Read the model definition and answer for the solid it produces. Units are mm, in the model's axes. A direction names the side the tool comes from. Round coordinates to 2 decimals unless told otherwise and drop trailing zeros. Write each loop counter-clockwise with the first axis right and the second up, starting at its lowest first coordinate (ties: lowest second). Pieces come first, ordered by that corner, then holes. Notation, with made-up numbers: (55, 0) - (109, 0) arc R26 cw to (109, 24) - close; hole circle Ø9 at (89.25, 45). An arc over 180 degrees is marked (long way). Answer as CSV lines item,"result". Start each with the question number.
1) Each of these flat-tipped pins is pushed along its axis until it touches: pin 1 (3 mm diameter, centred on x = -393, y = -7, fed in from -Z); pin 2 (5 mm diameter, centred on x = -390.5, y = -6.5, fed in from +Z); pin 3 (4 mm diameter, centred on x = -401.69, z = 27.68, fed in from -Y). Where does it stop, or does it pass through?
2) Find section B-B on y = 2. Determine the outline of the cut face in (x, z).
3) Consider line 1 along Z through (x, y) = (-394, -3.25); line 2 along X through (y, z) = (-7.75, 81.5); line 3 along Z through (x, y) = (-392.5, 2.25). Determine where each line is inside the solid, lowest interval first.
4) Which of the six approach directions +Z, -Z, +X, -X, +Y, -Y give full straight-line access (tool end or side, diameter ignored) to faces 4 (the flat face through (-402, -11, 69)), 5 (the flat face through (-392, -4, 70.38)), 6 (the cylindrical face through (-394.09, -10.4, 34.45)), 7 (the flat face through (-397, 1, 32.678)), 8 (the flat face through (-402, -4, 32.678))?
5) Find section C-C on y = -6.5. State how many separate pieces and enclosed holes the cut face has, then the cut area to 3 significant figures.
6) For a pull along X with two mould halves and no side action, classify faces 1 (the flat face through (-404.69, 1, 58)), 2 (the cylindrical face through (-389.942, 1.479, 28.218)), 3 (the flat face through (-397, 0, 89)) as +X half, -X half, draft (parallel to the pull), parting line (faces both ways), or undercut.
7) Find section A-A on z = 69.5. Determine the outline of the cut face in (x, y).
Autodesk Inventor part; units mm, degrees
ref_plane "工作平面4" through (-396.6746, 0, 58.7787) normal (1, 0, 0) x (0, 0, -1)
ref_plane "YZ Plane" through (0, 0, 0) normal (1, 0, 0) x (0, 1, 0)
ref_plane "XZ Plane" through (0, 0, 0) normal (0, 1, 0) x (-1, 0, 0)
sketch "草圖1" plane through (0, 0, 0) normal (0, 1, 0) x (-1, 0, 0)
  line L0 (403.4401, 81.3797) -> (399.9401, 81.3797) construction
  line L1 (399.9401, 81.3797) -> (399.9401, 70.3797) construction
  line L2 (399.9401, 70.3797) -> (403.4401, 70.3797) construction
  line L3 (403.4401, 70.3797) -> (403.4401, 81.3797) construction
  line L4 (403.4401, 81.3797) -> (399.9401, 70.3797) construction
  line L5 (399.9401, 81.3797) -> (403.4401, 70.3797) construction
  line L6 (403.4401, 70.3797) -> (404.6901, 70.3797)
  line L7 (398.6901, 70.3797) -> (403.4401, 70.3797)
  line L8 (403.4401, 81.3797) -> (404.6901, 81.3797)
  line L9 (404.6901, 84.8797) -> (398.6901, 84.8797)
  line L10 (398.6901, 81.3797) -> (403.4401, 81.3797)
  line L11 (404.6901, 93.8797) -> (398.6901, 93.8797)
  line L12 (398.6901, 93.8797) -> (398.6901, 57.8797)
  line L13 (404.6901, 57.8797) -> (404.6901, 93.8797)
  line L14 (404.6901, 93.8797) -> (398.6901, 57.8797) construction
  line L15 (398.6901, 93.8797) -> (404.6901, 57.8797) construction
  line L16 (401.6901, 84.8797) -> (401.6901, 89.8797) construction
  circle A0 centre (401.6901, 89.8797) radius 1.8
  line L17 (401.6901, 75.8797) -> (401.6901, 41.6777) construction
  circle A1 centre (401.6901, 58.7787) radius 1.8
  line L18 (404.6901, 66.8797) -> (398.6901, 66.8797)
  line L19 (403.4401, 36.1777) -> (399.9401, 36.1777) construction
  line L20 (399.9401, 36.1777) -> (399.9401, 47.1777) construction
  line L21 (399.9401, 47.1777) -> (403.4401, 47.1777) construction
  line L22 (403.4401, 47.1777) -> (403.4401, 36.1777) construction
  line L23 (403.4401, 36.1777) -> (399.9401, 47.1777) construction
  line L24 (399.9401, 36.1777) -> (403.4401, 47.1777) construction
  line L25 (403.4401, 47.1777) -> (404.6901, 47.1777)
  line L26 (398.6901, 47.1777) -> (403.4401, 47.1777)
  line L27 (403.4401, 36.1777) -> (404.6901, 36.1777)
  line L28 (404.6901, 32.6777) -> (398.6901, 32.6777)
  line L29 (398.6901, 36.1777) -> (403.4401, 36.1777)
  line L30 (404.6901, 23.6777) -> (398.6901, 23.6777)
  line L31 (398.6901, 23.6777) -> (398.6901, 59.6777)
  line L32 (404.6901, 59.6777) -> (404.6901, 23.6777)
  line L33 (404.6901, 23.6777) -> (398.6901, 59.6777) construction
  line L34 (398.6901, 23.6777) -> (404.6901, 59.6777) construction
  line L35 (401.6901, 32.6777) -> (401.6901, 27.6777) construction
  circle A2 centre (401.6901, 27.6777) radius 1.8
  circle A3 centre (401.6901, 58.7787) radius 1.8
  line L36 (404.6901, 50.6777) -> (398.6901, 50.6777)
  line L37 (404.6901, 66.8797) -> (398.6901, 66.8797)
  line L38 (398.6901, 66.8797) -> (398.6901, 50.6777)
  line L39 (398.6901, 50.6777) -> (404.6901, 50.6777)
  line L40 (404.6901, 50.6777) -> (404.6901, 66.8797)
  line L41 (401.6901, 58.7787) -> (391.6591, 58.7787) construction
  line L42 (396.6746, 58.7787) -> (396.6746, 63.5433) construction
  line L43 (391.6591, 58.7787) -> (401.6901, 58.7787) construction
  line L44 (398.6901, 66.8797) -> (394.6591, 66.8797)
  line L45 (398.6901, 50.6777) -> (394.6591, 50.6777)
  point P0 (0, 0)
  point P1 (398.1901, 70.3797)
  point P2 (398.1901, 81.3797)
  point P3 (398.1901, 47.1777)
  point P4 (398.1901, 36.1777)
  dimension "d8" = 11
  dimension "d34" = 36
  dimension "d35" = 5
  dimension "d37" = 3.6
  dimension "d49" = 34.202
  dimension "d50" = 3.6
  dimension "d61" = 10.031
extrude "擠出8" add sketch "草圖1" along normal blind 3
extrude "擠出9" add sketch "草圖1" against normal blind 11 contours L6 L13 L18 L12 L7 | L8 L10 L12 L9 L13 | L32 L25 L26 L31 L36 | L32 L28 L31 L29 L27
fillet "圓角4" radius 2 8 edges at (-404.6901, -11, 34.4277) (-398.6901, -11, 34.4277) (-404.6901, -11, 48.9277) (-398.6901, -11, 48.9277) (-404.6901, -11, 68.6297) (-398.6901, -11, 68.6297) (-398.6901, -11, 83.1297) (-404.6901, -11, 83.1297)
sketch "草圖4" plane through (-398.6901, 0, 32.6777) normal (0, 0, -1) x (-1, 0, 0)
  line L0 (0, 0) -> (6, 0) construction
  line L1 (6, 0) -> (3, 0) construction
  line L2 (3, 0) -> (3, -6.5) construction
  circle A0 centre (3, -6.5) radius 1.8
  point P0 (-398.6901, 0)
  dimension "d57" = 6.5
  dimension "d58" = 3.6
extrude "擠出10" cut sketch "草圖4" against normal through all
ref_plane "工作平面4" through (-396.6746, 0, 58.7787) normal (1, 0, 0) x (0, 0, -1)
mirror "鏡射2" about plane through (-396.6746, 0, 58.7787) normal (1, 0, 0) of "擠出8", "擠出9", "擠出10", "圓角4"
sketch "草圖8" plane through (0, 0, 0) normal (0, 1, 0) x (-1, 0, 0)
  line L0 (398.6901, 32.6777) -> (398.6901, 23.6777)
  line L1 (394.6591, 32.6777) -> (394.6591, 23.6777)
  line L2 (398.6901, 93.8797) -> (398.6901, 84.8797)
  line L3 (394.6591, 93.8797) -> (394.6591, 84.8797)
  line L4 (404.6901, 93.8797) -> (398.6901, 93.8797)
  line L5 (388.6591, 93.8797) -> (394.6591, 93.8797)
  line L6 (398.6901, 93.8797) -> (394.6591, 93.8797)
  line L7 (398.6901, 84.8797) -> (394.6591, 84.8797)
  line L8 (398.6901, 32.6777) -> (394.6591, 32.6777)
  line L9 (398.6901, 23.6777) -> (394.6591, 23.6777)
  point P0 (0, 0)
extrude "擠出13" add sketch "草圖8" along normal blind 3
properties part number "a臂鎖"
Check values:
1,pin 1,"stops at z = 32.68"
1,pin 2,"stops at z = 84.88"
1,pin 3,"stops at y = 0"
2,outline,"(-404.69, 23.68) - (-388.66, 23.68) - (-388.66, 93.88) - (-404.69, 93.88) - close; hole circle Ø3.6 at (-401.69, 27.68); hole circle Ø3.6 at (-401.69, 58.78); hole circle Ø3.6 at (-401.69, 89.88); hole (-398.69, 32.68) - (-394.66, 32.68) - (-394.66, 84.88) - (-398.69, 84.88) - close; hole circle Ø3.6 at (-391.66, 27.68); hole circle Ø3.6 at (-391.66, 58.78); hole circle Ø3.6 at (-391.66, 89.88)"
3,line 1,"z = 32.68 to 36.18, 47.18 to 50.68, 66.88 to 70.38, 81.38 to 84.88"
3,line 2,"x = -404.69 to -402.99, -400.39 to -398.69, -394.66 to -392.95, -390.36 to -388.66"
3,line 3,"z = 23.68 to 26.09, 29.27 to 57.19, 60.37 to 88.29, 91.47 to 93.88"
4,face 4,"+Z, -Z, +X, -X, -Y"
4,face 5,"+X, -X, -Y"
4,face 6,"+Z, -Z, -Y"
4,face 7,"+Y, -Y"
4,face 8,"-Z, +X, -X, -Y"
5,separate pieces,"16"
5,enclosed holes,"0"
5,area,"67.2 mm^2"
6,face 1,"-X half"
6,face 2,"undercut"
6,face 3,"draft"
7,outline,"(-404.69, -9) arc R2 ccw to (-402.69, -11) - (-400.69, -11) arc R2 ccw to (-398.69, -9) - (-398.69, 3) - (-404.69, 3) - close; (-394.66, -9) arc R2 ccw to (-392.66, -11) - (-390.66, -11) arc R2 ccw to (-388.66, -9) - (-388.66, 3) - (-394.66, 3) - close; hole circle Ø3.6 at (-401.69, -6.5); hole circle Ø3.6 at (-391.66, -6.5)"
